Autodesk Inventor part; units mm, degrees
ref_plane "YZ Plane" through (0, 0, 0) normal (1, 0, 0) x (0, 1, 0)
ref_plane "XZ Plane" through (0, 0, 0) normal (0, 1, 0) x (-1, 0, 0)
ref_plane "XY Plane" through (0, 0, 0) normal (0, 0, 1) x (1, 0, 0)
sketch "Náčrt1" plane through (0, 0, 0) normal (0, 0, 1) x (1, 0, 0)
  line L0 (-40, 10) -> (10, 10)
  line L1 (10, 10) -> (10, -10)
  line L2 (10, -10) -> (-40, -10)
  line L3 (-40, -10) -> (-40, 10)
  point P0 (0, 0)
  dimension "d0" = 20
  dimension "d1" = 50
  dimension "d2" = 10
  dimension "d3" = 10
extrude "Vysunutí1" add sketch "Náčrt1" along normal blind 0.5
sketch "Náčrt2" plane through (0, 0, 0.5) normal (0, 0, 1) x (1, 0, 0)
  circle A0 centre (-35, 5) radius 2
  line L0 (10, 10) -> (-40, 10)
  line L1 (-40, 10) -> (-40, -10)
  point P0 (0, 0)
  dimension "d6" = 4
  dimension "d7" = 5
  dimension "d8" = 5
extrude "Vysunutí2" cut sketch "Náčrt2" against normal blind 0.5
pattern_linear "Obdélníkové pole1" count 7 spacing 10 along (1, 0, 0) of "Vysunutí2"
fillet "Zaoblení1" radius 1 1 edges at (10, 10, 0.25)
fillet "Zaoblení2" radius 1 2 edges at (-40, 10, 0.25) (-40, -10, 0.25)
fillet "Zaoblení3" radius 1 1 edges at (10, -10, 0.25)
sketch "Náčrt3" plane through (0, 0, 0.5) normal (0, 0, 1) x (1, 0, 0)
  line L0 (7, -2.7639) -> (7, -7.2361)
  line L1 (3, -2.7639) -> (3, -7.2361)
  arc A0 (7, -2.7639) -> (3, -2.7639) centre (5, -5) ccw
  arc A1 (3, -7.2361) -> (7, -7.2361) centre (5, -5) ccw
  line L2 (10, -9) -> (10, 9)
  line L3 (-39, -10) -> (9, -10)
  point P0 (0, 0)
  point P1 (3, -7.229)
  point P2 (5, -8)
  point P3 (5, -2)
  dimension "d24" = 2
  dimension "d25" = 4
  dimension "d26" = 5
  dimension "d27" = 5
  dimension "d28" = 3
  dimension "d29" = 3
extrude "Vysunutí3" cut sketch "Náčrt3" against normal blind 10
pattern_linear "Obdélníkové pole2" count 7 spacing 10 along (-1, 0, 0) of "Vysunutí3"
properties part number "1020"
Input: part model. Units: mm. Frame: model coordinates. Give positions to 0.01 mm unless a question says otherwise; leave off trailing zeros. Loops run counter-clockwise (first coordinate to the right, second up) from the corner with the lowest first, then second, coordinate; pieces in that order, holes last. Notation, with made-up numbers: M -13,86.25 L 22,86.25 A22 cw 22,92.25 Z; hole C 30,-27.75 d2. An arc over 180 degrees is marked long. Use CSV: the item, a comma, the result in double quotes.
(1) Section D-D, the plane x = -33.5. Return loops of the section in (y, z).
Outcome:
outline,"M -10,0 L -7.6,0 L -7.6,0.5 L -10,0.5 Z; M -2.4,0 L 3.68,0 L 3.68,0.5 L -2.4,0.5 Z; M 6.32,0 L 10,0 L 10,0.5 L 6.32,0.5 Z"
(2) Material intervals for L1, parallel to Y at x = -35, z = 0.1; L2, parallel to X at y = -3, z = 0.1; L3, parallel to Y at x = -13.5, z = 0.1, sorted ascending. Write a range as [from, to].
Outcome:
L1,"y = [-10, -8], [-2, 3], [7, 10]"
L2,"x = [-40, -37], [-33, -27], [-23, -17], [-13, -7], [-3, 3], [7, 10]"
L3,"y = [-10, -7.6], [-2.4, 3.68], [6.32, 10]"
(3) Section B-B, the plane z = 0.4. Count the separate pieces of the cut face and the enclosed holes in it, plus the area to 3 significant figures.
Outcome:
separate pieces,"1"
enclosed holes,"10"
area,"826 mm²"
(4) Section A-A, the plane x = -25. Return loops of the section in (y, z).
Outcome:
outline,"M -10,0 L -8,0 L -8,0.5 L -10,0.5 Z; M -2,0 L 3,0 L 3,0.5 L -2,0.5 Z; M 7,0 L 10,0 L 10,0.5 L 7,0.5 Z"
(5) Pull-direction query (Y, two-part tool) for faces 1 (the face through (-15, 0, 0.5)), 2 (the face through (-6.998, 5.088, 0.254)), 3 (the face through (9.699, -9.715, 0.254)); classes: pulls with the +Y half, pulls with the -Y half, needs draft (parallel to the pull), parting line crosses it, or undercut.
Outcome:
face 1,"needs draft"
face 2,"undercut"
face 3,"pulls with the -Y half"
(6) Section C-C, the plane y = -5.5. Return loops of the section in (x, z).
Outcome:
outline,"M -40,0 L -37,0 L -37,0.5 L -40,0.5 Z; M -33,0 L -27,0 L -27,0.5 L -33,0.5 Z; M -23,0 L -17,0 L -17,0.5 L -23,0.5 Z; M -13,0 L -7,0 L -7,0.5 L -13,0.5 Z; M -3,0 L 3,0 L 3,0.5 L -3,0.5 Z; M 7,0 L 10,0 L 10,0.5 L 7,0.5 Z"
